For this review, take the finished solid that the model builds, in its own axes (mm). A direction names the side the tool comes from. Round coordinates to 2 decimals unless told otherwise and drop trailing zeros. Loops run counter-clockwise (first coordinate to the right, second up) from the corner with the lowest first, then second, coordinate; pieces in that order, holes last.
1) Wall thickness on L1, parallel to X at y = 7.5, z = 0; L2, parallel to X at y = 2.8, z = 0; L3, parallel to Y at x = -8, z = -10: over which ranges is each line inside the solid? List them lowest first.
2) Take a section at B-B (x = 0). State the section outline as (y, z) points, then the cut area to 3 significant figures.
3) Tool access review of faces 4 (the flat face through (-11, 4, 1)), 5 (the cylindrical face through (-14.04, 5.07, 0.806)): name each direction out of +Z, -Z, +X, -X, +Y, -Y from which nothing blocks a thin tool from reaching the whole face with its end or side.
4) Take a section at D-D (x = 5). State the section outline as (y, z) points.
5) Take a section at C-C (z = -4). State the section outline as (x, y) points, then the cut area to 3 significant figures.
6) Take a section at A-A (z = 0). State the section outline as (x, y) points.
7) Mouldability with a two-part tool opening along X and no side actions: class faces 1 (the cylindrical face through (-11.56, 4.93, -15.08)), 2 (the cylindrical face through (-13.18, 1.97, 2.93)), 3 (the flat face through (4.5, 0, -12.9)) as pulls with the +X half, pulls with the -X half, needs draft (parallel to the pull), parting line crosses it, or undercut.
8) Insertion check: pin 1 (1 mm diameter, centred on x = 10.5, y = 5, fed in from -Z); pin 2 (6 mm diameter, centred on y = 7.5, z = 2, fed in from -X); pin 3 (1.5 mm diameter, centred on y = 5, z = 10, fed in from +X). Each pin has a flat end and moves straight along its axis. Give the tip position at first contact, or say it passes through.
```python
from build123d import *

# Parameters (mm, degrees)
SKETCH1_R          = 19
SKETCH1_R_2        = 10.75
EXTRUDE1_DEPTH     = 10
SKETCH2_R          = 13.5
CUT_EXTRUDE1_DEPTH = 4
SKETCH3_R          = 1.5
CUT_EXTRUDE2_DEPTH = 29.670542374


with BuildPart() as part:
    # Sketch1 → Extrude1 (new body)
    with BuildSketch(Plane(origin=(0, 0, 0), x_dir=(1, 0, 0), z_dir=(0, 1, 0))):
        with Locations(Location((0, 0, 0), (0, 0, 270))):
            Circle(SKETCH1_R)
        with Locations(Location((0, 0, 0), (0, 0, 270))):
            Circle(SKETCH1_R_2, mode=Mode.SUBTRACT)
    extrude(amount=EXTRUDE1_DEPTH)

    # Sketch2 → Cut-Extrude1 (cut)
    with BuildSketch(Plane.XZ):
        with Locations(Location((0, 0, 0), (0, 0, 270))):
            Circle(SKETCH2_R)
    extrude(amount=-CUT_EXTRUDE1_DEPTH, mode=Mode.SUBTRACT)

    # Sketch3 → Cut-Extrude2 (cut, through all)
    with BuildSketch(Plane(origin=(0, 10, 0), x_dir=(1, 0, 0), z_dir=(0, 1, 0))):
        with Locations(Location((0, 15.305022153, 0), (0, 0, 270))):
            Circle(SKETCH3_R)
        with Locations(Location((15.305022153, 0, 0), (0, 0, 270))):
            Circle(SKETCH3_R)
        with Locations(Location((0, -15.305022153, 0), (0, 0, 270))):
            Circle(SKETCH3_R)
        with Locations(Location((-15.305022153, 0, 0), (0, 0, 270))):
            Circle(SKETCH3_R)
    extrude(amount=-CUT_EXTRUDE2_DEPTH, mode=Mode.SUBTRACT)


solid = part.part
```
Response:
1. L1: x = -19 to -16.81, -13.81 to -10.75, 10.75 to 13.81, 16.81 to 19
1. L2: x = -19 to -16.81, -13.81 to -13.5, 13.5 to 13.81, 16.81 to 19
1. L3: y = 4 to 10
2. outline: (0, -19) - (10, -19) - (10, -16.81) - (0, -16.81) - close; (0, -13.81) - (10, -13.81) - (10, -10.75) - (4, -10.75) - (4, -13.5) - (0, -13.5) - close; (0, 13.5) - (4, 13.5) - (4, 10.75) - (10, 10.75) - (10, 13.81) - (0, 13.81) - close; (0, 16.81) - (10, 16.81) - (10, 19) - (0, 19) - close
2. area: 83.0 mm2
3. face 4: -Y
3. face 5: +Y, -Y
4. outline: (0, -18.33) - (10, -18.33) - (10, -9.52) - (4, -9.52) - (4, -12.54) - (0, -12.54) - close; (0, 12.54) - (4, 12.54) - (4, 9.52) - (10, 9.52) - (10, 18.33) - (0, 18.33) - close
5. outline: (-18.57, 0) - (-12.89, 0) - (-12.89, 4) - (-9.98, 4) - (-9.98, 10) - (-18.57, 10) - close; (9.98, 4) - (12.89, 4) - (12.89, 0) - (18.57, 0) - (18.57, 10) - (9.98, 10) - close
5. area: 149 mm2
6. outline: (-19, 0) - (-16.81, 0) - (-16.81, 10) - (-19, 10) - close; (-13.81, 0) - (-13.5, 0) - (-13.5, 4) - (-10.75, 4) - (-10.75, 10) - (-13.81, 10) - close; (10.75, 4) - (13.5, 4) - (13.5, 0) - (13.81, 0) - (13.81, 10) - (10.75, 10) - close; (16.81, 0) - (19, 0) - (19, 10) - (16.81, 10) - close
7. face 1: parting line crosses it
7. face 2: undercut
7. face 3: needs draft
8. pin 1: stops at z = -16.16
8. pin 2: stops at x = -19
8. pin 3: stops at x = 16.6
